Drawing for the job (mm, zero at the part's lowest x, y, z). Round coordinates to 2 decimals unless told otherwise and drop trailing zeros. Loops run counter-clockwise (first coordinate to the right, second up) from the corner with the lowest first, then second, coordinate; pieces in that order, holes last. Notation, with made-up numbers: M 16.5,62 L 63.5,62 A16 cw 63.5,71 Z; hole C 1.25,-14 d3. An arc over 180 degrees is marked long. Write each question's results on one line, items separated by ' | '.
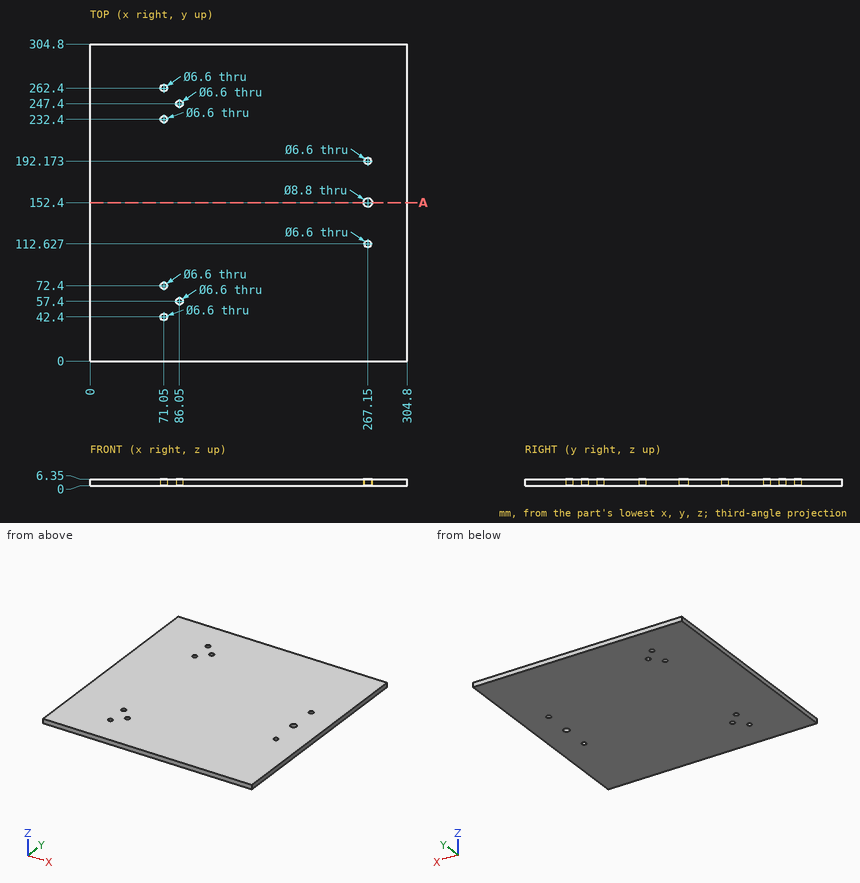
Item 1: Drop a flat-ended pin along its axis: P1, Ø7.5, axis at x = 71.05, y = 262.4, coming from the +Z side. Give the stop position or say it passes through.
Filled sheet:
P1: z = 6.35
Item 2: Band-saw the part on A-A on y = 152.4. Give the cut face in (x, z), and give its area (3 significant figures).
Filled sheet:
outline: M 0,0 L 262.75,0 L 262.75,6.35 L 0,6.35 Z; M 271.55,0 L 304.8,0 L 304.8,6.35 L 271.55,6.35 Z | area: 1,880 mm^2
Item 3: Wall check: L1, parallel to Y at x = 71.05, z = 3; L2, parallel to Y at x = 267.15, z = 3; L3, parallel to X at y = 262.4, z = 2.5. Give the ranges that are in metal, low to high.
Filled sheet:
L1: 0 to 39.1, 45.7 to 69.1, 75.7 to 229.1, 235.7 to 259.1, 265.7 to 304.8 | L2: 0 to 109.33, 115.93 to 148, 156.8 to 188.87, 195.47 to 304.8 | L3: 0 to 67.75, 74.35 to 304.8
